CAD build for the part. Positions are in the model's coordinates, mm. Coordinates: 2 decimals unless noted, no trailing zeros. Write each loop counter-clockwise with the first axis right and the second up, starting at its lowest first coordinate (ties: lowest second). Pieces come first, ordered by that corner, then holes. Notation, with made-up numbers: (5.25, 6.25) - (39.25, 6.25) arc R20 cw to (39.25, 31.25) - close; hole circle Ø2 at (75, 15.25). An arc over 180 degrees is marked (long way). Answer in a Markdown table with one row per item. Add a question column.
Q1. Band-saw the part on D-D (y = 149.5). List the corners of the cut face in (x, z).
Q2. Drill centre lines: line 1 along Y through (x, z) = (67, -0.55); line 2 along X through (y, z) = (19, -2.4); line 3 along Y through (x, z) = (54, -3.55). Where is each one in solid material? Low to high. Write a range as from..to.
Q3. Band-saw the part on C-C (x = 107.5). List the corners of the cut face in (y, z), and give its area (3 significant figures).
Q4. Band-saw the part on A-A (x = 45.5). List the corners of the cut face in (y, z).
Q5. Band-saw the part on B-B (y = 22). List the corners of the cut face in (x, z).
Q6. Pin check, flat tips, straight feed: pin 1 (1.2 mm diameter, centred on y = 150, z = -1, fed in from -X); pin 2 (2 mm diameter, centred on x = 24, z = -2, fed in from +Y); pin 3 (1.2 mm diameter, centred on x = 98.5, z = -2.5, fed in from -Y). Stop position of each tip, or through.
```python
from build123d import *

# Parameters (mm, degrees)
BUITENAFMETING_RECHTHOEK_W  = 130
BUITENAFMETING_RECHTHOEK_H  = 190
PLAAT_DEPTH                 = 4
TAND_HOR_W                  = 18.571428572
TAND_HOR_H                  = 4
TAND_BOVEN_DEPTH            = 5
TANDEN_PATROON_BOVEN_COUNT  = 3
TANDEN_PATROON_BOVEN_PITCH  = 37.142857143
TAND_VER_W                  = 4
TAND_VER_H                  = 27.142857143
TAND_LINKS_DEPTH            = 5
TANDEN_PATROON_LINKS_COUNT  = 3
TANDEN_PATROON_LINKS_PITCH  = 54.285714286
TAND_O_W                    = 18.571428572
TAND_O_H                    = 4
TAND_ONDER_DEPTH            = 5
TANDEN_PATROON_ONDER_COUNT  = 3
TANDEN_PATROON_ONDER_PITCH  = 37.142857143
TAND_R_W                    = 4
TAND_R_H                    = 27.142857143
TAND_RECHTS_DEPTH           = 5
TANDEN_PATROON_RECHTS_COUNT = 3
TANDEN_PATROON_RECHTS_PITCH = 54.285714286
SKETCH1_W                   = 80
SKETCH1_H                   = 35
CUT_EXTRUDE1_DEPTH          = 10


with BuildPart() as part:
    # Buitenafmeting Rechthoek → Plaat (new body)
    with BuildSketch(Plane.XY):
        with Locations((65, 95)):
            Rectangle(BUITENAFMETING_RECHTHOEK_W, BUITENAFMETING_RECHTHOEK_H)
    extrude(amount=-PLAAT_DEPTH)

    # Tand Hor → Tand Boven (cut, through all)
    with BuildSketch(Plane.XY):
        with Locations((27.857142857, 188)):
            Rectangle(TAND_HOR_W, TAND_HOR_H)
    tand_boven = extrude(amount=-TAND_BOVEN_DEPTH, mode=Mode.SUBTRACT)

    # Tanden Patroon Boven: Tand Boven ×3
    with Locations(*[(i * TANDEN_PATROON_BOVEN_PITCH, 0, 0) for i in range(1, TANDEN_PATROON_BOVEN_COUNT)]):
        add(tand_boven, mode=Mode.SUBTRACT)

    # Tand Ver → Tand Links (cut, through all)
    with BuildSketch(Plane.XY):
        with Locations((2, 149.285714286)):
            Rectangle(TAND_VER_W, TAND_VER_H)
    tand_links = extrude(amount=-TAND_LINKS_DEPTH, mode=Mode.SUBTRACT)

    # Tanden Patroon Links: Tand Links ×3
    with Locations(*[(0, -i * TANDEN_PATROON_LINKS_PITCH, 0) for i in range(1, TANDEN_PATROON_LINKS_COUNT)]):
        add(tand_links, mode=Mode.SUBTRACT)

    # Tand O → Tand Onder (cut, through all)
    with BuildSketch(Plane.XY):
        with Locations((27.857142857, 2)):
            Rectangle(TAND_O_W, TAND_O_H)
    tand_onder = extrude(amount=-TAND_ONDER_DEPTH, mode=Mode.SUBTRACT)

    # Tanden Patroon Onder: Tand Onder ×3
    with Locations(*[(i * TANDEN_PATROON_ONDER_PITCH, 0, 0) for i in range(1, TANDEN_PATROON_ONDER_COUNT)]):
        add(tand_onder, mode=Mode.SUBTRACT)

    # Tand R → Tand Rechts (cut, through all)
    with BuildSketch(Plane.XY):
        with Locations((128, 149.285714286)):
            Rectangle(TAND_R_W, TAND_R_H)
    tand_rechts = extrude(amount=-TAND_RECHTS_DEPTH, mode=Mode.SUBTRACT)

    # Tanden Patroon Rechts: Tand Rechts ×3
    with Locations(*[(0, -i * TANDEN_PATROON_RECHTS_PITCH, 0) for i in range(1, TANDEN_PATROON_RECHTS_COUNT)]):
        add(tand_rechts, mode=Mode.SUBTRACT)

    # Sketch1 → Cut-Extrude1 (cut)
    with BuildSketch(Plane.XY):
        with Locations((65, 29)):
            Rectangle(SKETCH1_W, SKETCH1_H)
    extrude(amount=-CUT_EXTRUDE1_DEPTH, mode=Mode.SUBTRACT)


solid = part.part
```
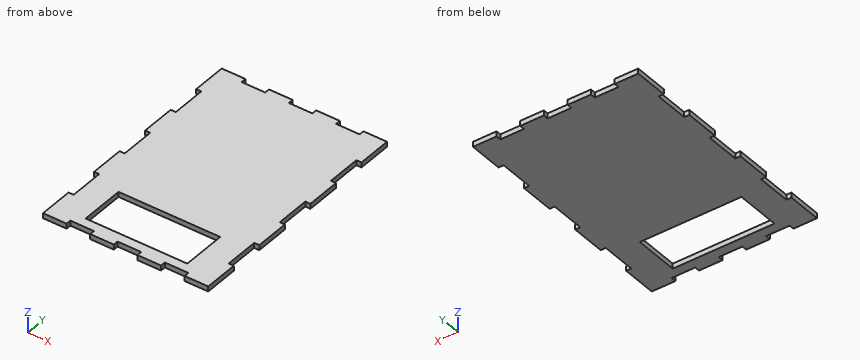
Checked values:
| question | item | result |
|---|---|---|
| 1 | outline | (4, -4) - (126, -4) - (126, 0) - (4, 0) - close |
| 2 | line 1 | y = 4..11.5, 46.5..186 |
| 2 | line 2 | x = 0..25, 105..130 |
| 2 | line 3 | y = 0..11.5, 46.5..190 |
| 3 | outline | (4, -4) - (186, -4) - (186, 0) - (4, 0) - close |
| 3 | area | 728 mm² |
| 4 | outline | (0, -4) - (11.5, -4) - (11.5, 0) - (0, 0) - close; (46.5, -4) - (190, -4) - (190, 0) - (46.5, 0) - close |
| 5 | outline | (0, -4) - (25, -4) - (25, 0) - (0, 0) - close; (105, -4) - (130, -4) - (130, 0) - (105, 0) - close |
| 6 | pin 1 | stops at x = 4 |
| 6 | pin 2 | stops at y = 186 |
| 6 | pin 3 | stops at y = 4 |
